from build123d import *

# Parameters (mm, degrees)
BOSS_EXTRUDE1_DEPTH = 3.175
SKETCH2_W           = 150
SKETCH2_H           = 50
CUT_EXTRUDE1_DEPTH  = 10


with BuildPart() as part:
    # Sketch1 → Boss-Extrude1 (new body)
    with BuildSketch(Plane(origin=(0, 0, 0), x_dir=(1, 0, 0), z_dir=(0, 1, 0))):
        Polygon((-175, 100), (175, 100), (275, 0), (200, -500), (-200, -500), (-275, 0), align=None)
    extrude(amount=BOSS_EXTRUDE1_DEPTH)

    # Sketch2 → Cut-Extrude1 (cut)
    with BuildSketch(Plane(origin=(0, 3.175, 0), x_dir=(1, 0, 0), z_dir=(0, 1, 0))):
        with Locations((0, -205)):
            Rectangle(SKETCH2_W, SKETCH2_H)
        with Locations((0, -125)):
            Rectangle(SKETCH2_W, SKETCH2_H)
    extrude(amount=-CUT_EXTRUDE1_DEPTH, mode=Mode.SUBTRACT)


solid = part.part
The listing builds one solid part. Answer for the finished solid, in the listing's coordinates (mm). Give positions to 0.01 mm unless a question says otherwise; leave off trailing zeros. Write each loop counter-clockwise with the first axis right and the second up, starting at its lowest first coordinate (ties: lowest second). Pieces come first, ordered by that corner, then holes.
1) Section B-B (y = 1.1) is taken. Write down the section's boundary in (x, z).
2) Section D-D (x = 193) is taken. Write down the section's boundary in (y, z) (3 decimals).
3) Section A-A (x = 8.5) is taken. Write down the section's boundary in (y, z) (3 decimals), and give its area (3 significant figures).
4) Given P1, Ø1, axis at y = 2, z = 135.5, coming from the +X side, flat-ended and moving along its own axis, determine where the tip first touches the part or whether it passes through.
5) Find the intervals of material crossed by L1, parallel to Z at x = 1.5, y = 2.65; L2, parallel to X at y = 3.05, z = 130; L3, parallel to X at y = 2.4, z = 196, in increasing order.
6) Section C-C (z = 384) is taken. Write down the section's boundary in (x, y) (3 decimals), and give its area (3 significant figures).
Response:
1. outline: (-275, 0) - (-175, -100) - (175, -100) - (275, 0) - (200, 500) - (-200, 500) - close; hole (-75, 100) - (75, 100) - (75, 150) - (-75, 150) - close; hole (-75, 180) - (75, 180) - (75, 230) - (-75, 230) - close
2. outline: (0, -82) - (3.175, -82) - (3.175, 500) - (0, 500) - close
3. outline: (0, -100) - (3.175, -100) - (3.175, 100) - (0, 100) - close; (0, 150) - (3.175, 150) - (3.175, 180) - (0, 180) - close; (0, 230) - (3.175, 230) - (3.175, 500) - (0, 500) - close
3. area: 1,590 mm2
4. P1: stops at x = 254.75
5. L1: z = -100 to 100, 150 to 180, 230 to 500
5. L2: x = -255.5 to -75, 75 to 255.5
5. L3: x = -245.6 to -75, 75 to 245.6
6. outline: (-217.4, 0) - (217.4, 0) - (217.4, 3.175) - (-217.4, 3.175) - close
6. area: 1,380 mm2
